Drawing for the job (mm, zero at the part's lowest x, y, z). Give positions to 0.01 mm unless a question says otherwise; leave off trailing zeros. Loops run counter-clockwise (first coordinate to the right, second up) from the corner with the lowest first, then second, coordinate; pieces in that order, holes last. Notation, with made-up numbers: M 84.25,80.25 L 132.25,80.25 A16 cw 132.25,94.25 Z; hole C 83,-19.75 d1. An arc over 180 degrees is marked long. Use CSV: the item, a comma, the result in double quotes. Start each with the question number.
(1) Slice it at B-B on x = 14. List the corners of the cut face in (y, z) (1 decimal).
(2) Slice it at C-C on z = 1.05. List the corners of the cut face in (x, y) (1 decimal).
(3) Two-plate mould, pull along Y, no slides. Class the marked faces 1, 2, 3 and 4: pulls with the +Y half, pulls with the -Y half, needs draft (parallel to the pull), parting line crosses it, or undercut.
(4) Flat gauge pins, fed straight in: P1, Ø3.5, axis at x = 20.66, y = 4.66, coming from the -Z side; P2, Ø1, axis at y = 11, z = 2.5, coming from the -X side. Where does each tip first touch, or does it go through?
(5) Slice it at A-A on y = 36. List the corners of the cut face in (x, z).
(6) Wall check: line 1 along X through (y, z) = (22, 0.55) (1 decimal); line 2 along Y through (x, z) = (21.5, 2.9) (1 decimal). Give the ranges that are in metal, low to high. Write a range as from..to.
(7) Slice it at D-D on y = 7. List the corners of the cut face in (x, z).
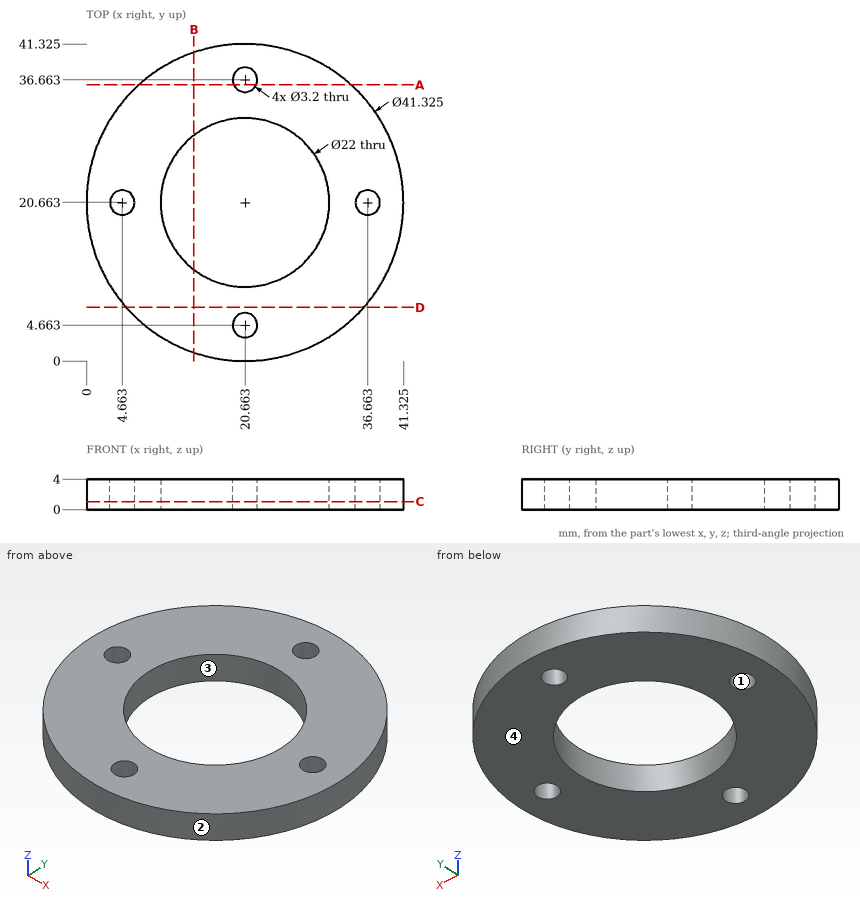
Reply:
1,outline,"M 1.1,0 L 11.9,0 L 11.9,4 L 1.1,4 Z; M 29.4,0 L 40.2,0 L 40.2,4 L 29.4,4 Z"
2,outline,"C 20.7,20.7 d41.3; hole C 4.7,20.7 d3.2; hole C 20.7,20.7 d22; hole C 20.7,4.7 d3.2; hole C 20.7,36.7 d3.2; hole C 36.7,20.7 d3.2"
3,face 1,"undercut"
3,face 2,"parting line crosses it"
3,face 3,"undercut"
3,face 4,"needs draft"
4,P1,"stops at z = 0"
4,P2,"stops at x = 2.14"
5,outline,"M 6.82,0 L 19.21,0 L 19.21,4 L 6.82,4 Z; M 22.12,0 L 34.51,0 L 34.51,4 L 22.12,4 Z"
6,line 1,"x = 0..3.8, 5.5..9.7, 31.6..35.8, 37.5..41.3"
6,line 2,"y = 0..3.3, 6..9.7, 31.6..35.3, 38..41.3"
7,outline,"M 5.16,0 L 36.16,0 L 36.16,4 L 5.16,4 Z"
